from build123d import *

# Parameters (mm, degrees)
SKETCH1_W           = 76.560291348
SKETCH1_H           = 108.5
SKETCH1_R           = 3.2639
BOSS_EXTRUDE1_DEPTH = 8.4
SKETCH1_3_W         = 35
SKETCH1_3_H         = 48.7
SKETCH1_3_R         = 3.2639
BOSS_EXTRUDE2_DEPTH = 8.9
SKETCH1_4_W         = 76.560291348
SKETCH1_4_H         = 32.3
BOSS_EXTRUDE3_DEPTH = 10
FILLET1_R           = 3
CHAMFER1_SIZE       = 0.5


with BuildPart() as part:
    # Sketch1 → Boss-Extrude1 (new body)
    with BuildSketch(Plane.XY):
        with Locations((83.619854326, -16.15)):
            Rectangle(SKETCH1_W, SKETCH1_H)
        with Locations((104.4, -14.4)):
            Circle(SKETCH1_R, mode=Mode.SUBTRACT)
    extrude(amount=BOSS_EXTRUDE1_DEPTH)

    # Sketch1<3> → Boss-Extrude2 (add)
    with BuildSketch(Plane.XY):
        with Locations((104.4, -13.75)):
            Rectangle(SKETCH1_3_W, SKETCH1_3_H)
        with Locations((104.4, -14.4)):
            Circle(SKETCH1_3_R, mode=Mode.SUBTRACT)
    extrude(amount=BOSS_EXTRUDE2_DEPTH)

    # Sketch1<4> → Boss-Extrude3 (add)
    with BuildSketch(Plane.XY):
        with Locations((83.619854326, -54.25)):
            Rectangle(SKETCH1_4_W, SKETCH1_4_H)
    extrude(amount=-BOSS_EXTRUDE3_DEPTH)

    # Fillet1
    fillet1_edges = [part.edges().sort_by_distance(p)[0] for p in [
        (45.339708652, 38.1, 4.2),
        (121.9, -38.1, 8.65),
        (86.9, -38.1, 8.65),
        (86.9, 10.6, 8.65),
        (121.9, 10.6, 8.65),
        (45.339708652, -70.4, -0.8),
        (121.9, -38.1, -5),
        (45.339708652, -38.1, -5),
        (121.9, -70.4, -0.8),
        (121.9, 38.1, 4.2),
    ]]
    fillet(fillet1_edges, radius=FILLET1_R)

    # Chamfer1
    chamfer1_edges = [part.edges().sort_by_distance(p)[0] for p in [
        (121.9, 22.85, 8.4),
        (101.1361, -14.4, 8.9),
        (101.1361, -14.4, 0),
        (121.9, -54.25, -10),
        (121.9, -1.5, 0),
        (121.9, -52.75, 8.4),
        (45.339708652, -16.15, 8.4),
        (45.339708652, -1.5, 0),
        (45.339708652, -54.25, -10),
        (83.619854326, 38.1, 0),
        (121.021320344, 37.221320344, 0),
        (46.218388308, 37.221320344, 0),
        (83.619854326, 38.1, 8.4),
        (83.619854326, -70.4, 8.4),
        (121.021320344, -69.521320344, 8.4),
        (46.218388308, -69.521320344, 8.4),
        (121.021320344, 37.221320344, 8.4),
        (46.218388308, 37.221320344, 8.4),
        (83.619854326, -38.1, -10),
        (83.619854326, -70.4, -10),
        (121.021320344, -69.521320344, -10),
        (46.218388308, -69.521320344, -10),
        (121.021320344, -38.978679656, -10),
        (46.218388308, -38.978679656, -10),
    ]]
    chamfer(chamfer1_edges, length=CHAMFER1_SIZE)


solid = part.part
Geometry: final body of the model. Coordinates: model frame, mm. A direction names the side the tool comes from. Give positions to 0.01 mm unless a question says otherwise; leave off trailing zeros. Loops run counter-clockwise (first coordinate to the right, second up) from the corner with the lowest first, then second, coordinate; pieces in that order, holes last. Notation, with made-up numbers: (-20.5, 34) - (33.5, 34) arc R17 ccw to (33.5, 41) - close; hole circle Ø1 at (-25, -5). An arc over 180 degrees is marked (long way). Answer as CSV lines item,"result". Start each with the question number.
1. Section B-B, the plane y = -14.4. Return loops of the section in (x, z), plus the area to 3 significant figures.
2. Section D-D, the plane y = -59. Return loops of the section in (x, z), plus the area to 3 significant figures.
3. Reachability of faces 1 (the face through (121.04, -39, -4.57)), 2 (the face through (83, 0, 0)), 3 (the face through (87.8, -37.24, 8.65)), 4 (the face through (121.338, -36.848, 8.629)) from +Z, -Z, +X, -X, +Y, -Y: full face, straight path, thin tool, end or side. Return the list, or none.
4. Section A-A, the plane x = 104.4. Return loops of the section in (y, z), plus the area to 3 significant figures.
5. Pin query (flat end, axial travel): P1, Ø6, axis at x = 104.4, y = -14.4, coming from the -Z side; P2, Ø3, axis at x = 96.5, z = -4.5, coming from the +Y side; P3, Ø1.5, axis at x = 56, y = 12, coming from the +Z side; P4, Ø0.6, axis at x = 100.5, z = 8.5, coming from the +Y side. Return the tip coordinate at first contact, or that it passes through.
6. Section C-C, the plane z = -7.25. Return loops of the section in (x, y), plus the area to 3 significant figures.
7. Ray query, L1, parallel to Y at x = 104.4, z = 6.5; L2, parallel to Y at x = 78, z = -5.5; L3, parallel to Z at x = 82, y = -5. Return the intervals inside material, ascending.
Answers:
1,outline,"(45.34, 0.5) - (45.84, 0) - (100.64, 0) - (101.14, 0.5) - (101.14, 8.4) - (100.64, 8.9) - (86.9, 8.9) - (86.9, 8.4) - (45.84, 8.4) - (45.34, 7.9) - close; (107.66, 0.5) - (108.16, 0) - (121.4, 0) - (121.9, 0.5) - (121.9, 8.9) - (108.16, 8.9) - (107.66, 8.4) - close"
1,area,"602 mm2"
2,outline,"(45.34, -9.5) - (45.84, -10) - (121.4, -10) - (121.9, -9.5) - (121.9, 7.9) - (121.4, 8.4) - (45.84, 8.4) - (45.34, 7.9) - close"
2,area,"1,410 mm2"
3,face 1,"-Z, +X, +Y"
3,face 2,"-Z, +X, -X, +Y"
3,face 3,"+Z, -X, -Y"
3,face 4,"+Z, +X, -Y"
4,outline,"(-70.4, -9.5) - (-69.9, -10) - (-38.6, -10) - (-38.1, -9.5) - (-38.1, 0) - (-18.16, 0) - (-17.66, 0.5) - (-17.66, 8.4) - (-18.16, 8.9) - (-38.1, 8.9) - (-38.1, 8.4) - (-69.9, 8.4) - (-70.4, 7.9) - close; (-11.14, 0.5) - (-10.64, 0) - (37.6, 0) - (38.1, 0.5) - (38.1, 7.9) - (37.6, 8.4) - (10.6, 8.4) - (10.6, 8.9) - (-10.64, 8.9) - (-11.14, 8.4) - close"
4,area,"1,200 mm2"
5,P1,"passes through"
5,P2,"stops at y = -38.1"
5,P3,"stops at z = 8.4"
5,P4,"stops at y = 37.8"
6,outline,"(45.34, -67.4) arc R3 ccw to (48.34, -70.4) - (118.9, -70.4) arc R3 ccw to (121.9, -67.4) - (121.9, -41.1) arc R3 ccw to (118.9, -38.1) - (48.34, -38.1) arc R3 ccw to (45.34, -41.1) - close"
6,area,"2,470 mm2"
7,L1,"y = -70.4 to -17.66, -11.14 to 38.1"
7,L2,"y = -70.4 to -38.1"
7,L3,"z = 0 to 8.4"
